```python
from build123d import *

# Parameters (mm, degrees)
SKETCH1_R           = 2
BOSS_EXTRUDE1_DEPTH = 1.5


with BuildPart() as part:
    # Sketch1 → Boss-Extrude1 (new body, symmetric)
    with BuildSketch(Plane.XY):
        with BuildLine():
            Line((0, 88.5), (-2, 86.5))
            Line((-2, 86.5), (0, 84.5))
            Line((0, 84.5), (-2, 82.5))
            Line((-2, 82.5), (0, 80.5))
            Line((0, 80.5), (-2, 78.5))
            Line((-2, 78.5), (0, 76.5))
            Line((0, 76.5), (0, 75))
            ThreePointArc((0, 75), (-5.309927761, 63.55), (0, 52.1))
            Line((0, 52.1), (-2, 50.1))
            Line((-2, 50.1), (0, 48.1))
            Line((0, 48.1), (-2, 46.1))
            Line((-2, 46.1), (0, 44.1))
            Line((0, 44.1), (-2, 42.1))
            ThreePointArc((-2, 42.1), (-4.035298286, 39.053960857), (-4.75, 35.460912703))
            Line((-4.75, 35.460912703), (-4.75, 0))
            ThreePointArc((-4.75, 0), (-11.25, -6.5), (-17.75, 0))
            Line((-17.75, 0), (-17.75, 67.916352203))
            Line((-17.75, 67.916352203), (-5, 90))
            Line((-5, 90), (0, 90))
            Line((0, 90), (0, 88.5))
        make_face()
        with Locations((-9.75, 0)):
            Circle(SKETCH1_R, mode=Mode.SUBTRACT)
        with Locations((-9.75, 25)):
            Circle(SKETCH1_R, mode=Mode.SUBTRACT)
    extrude(amount=BOSS_EXTRUDE1_DEPTH, both=True)


solid = part.part
```
Here's how the part is built. I have some questions about the finished solid (model axes, mm). A direction names the side the tool comes from. Give positions to 0.01 mm unless a question says otherwise; leave off trailing zeros. Order: outer loops, then holes, each group sorted by start corner. A loop starts at its lowest first (then second) coordinate and runs counter-clockwise, first axis right, second up. Notation, with made-up numbers: M 20,-6 L 79,-6 A30 cw 79,25 Z; hole C 69,54 d8. An arc over 180 degrees is marked long. Use a Markdown table: item, result. Add a question column.
1. Suppose I cut it at B-B (z = 0.85). List the corners of the cut face in (x, y) for me.
2. On a 3-axis mill with a long thin cutter (end or side, diameter ignored), from which of +Z, -Z, +X, -X, +Y, -Y can I reach the whole of each face in a straight line? I mean faces 1 (the flat face through (-1, 43.1, 0)), 2 (the flat face through (-1, 83.5, 0)). Say none if no direction works.
3. Suppose I cut it at C-C (x = -9.75). List the corners of the cut face in (y, z) for me, and give its area (3 significant figures).
4. If we mould it in two halves opening along X, with no side actions, what happens to faces 3 (the flat face through (-17.75, 33, 0)), 4 (the cylindrical face through (-10.184, 23.048, -0.021)), 5 (the flat face through (-1, 85.5, 0))? For each: +X half, -X half, draft (parallel to the pull), parting line (faces both ways), or undercut.
5. Suppose I cut it at D-D (x = -16.25). List the corners of the cut face in (y, z) for me.
6. I need wall thicknesses on probe 1 along Y at (x, z) = (-9.75, -0.4); probe 2 along X at (y, z) = (17.5, -0.35); probe 3 along Y at (x, z) = (-2.5, 0.35). Which ranges of each line are inside material? Lowest first, please. Write a range as from..to.
7. Suppose I cut it at A-A (y = 25). List the corners of the cut face in (x, z) for me.
Results list:
| question | item | result |
|---|---|---|
| 1 | outline | M -17.75,0 A6.5 ccw -4.75,0 L -4.75,35.46 A9.39 cw -2,42.1 L 0,44.1 L -2,46.1 L 0,48.1 L -2,50.1 L 0,52.1 A15 cw 0,75 L 0,76.5 L -2,78.5 L 0,80.5 L -2,82.5 L 0,84.5 L -2,86.5 L 0,88.5 L 0,90 L -5,90 L -17.75,67.92 Z; hole C -9.75,0 d4; hole C -9.75,25 d4 |
| 2 | face 1 | +Z, -Z, +X, -Y |
| 2 | face 2 | +Z, -Z, +X |
| 3 | outline | M -6.32,-1.5 L -2,-1.5 L -2,1.5 L -6.32,1.5 Z; M 2,-1.5 L 23,-1.5 L 23,1.5 L 2,1.5 Z; M 27,-1.5 L 81.77,-1.5 L 81.77,1.5 L 27,1.5 Z |
| 3 | area | 240 mm² |
| 4 | face 3 | -X half |
| 4 | face 4 | undercut |
| 4 | face 5 | +X half |
| 5 | outline | M -4.15,-1.5 L 70.51,-1.5 L 70.51,1.5 L -4.15,1.5 Z |
| 6 | probe 1 | y = -6.32..-2, 2..23, 27..81.77 |
| 6 | probe 2 | x = -17.75..-4.75 |
| 6 | probe 3 | y = 41.56..54.81, 72.29..90 |
| 7 | outline | M -17.75,-1.5 L -11.75,-1.5 L -11.75,1.5 L -17.75,1.5 Z; M -7.75,-1.5 L -4.75,-1.5 L -4.75,1.5 L -7.75,1.5 Z |
